Could you check a few things on this model? Use its own coordinates, in mm. A direction names the side the tool comes from. Give positions to 0.01 mm unless a question says otherwise; leave off trailing zeros. Order: outer loops, then holes, each group sorted by start corner. A loop starts at its lowest first (then second) coordinate and runs counter-clockwise, first axis right, second up. Notation, with made-up numbers: M 59,-5 L 66,-5 A8 cw 66,1 Z; hole C 84.25,56.5 d8. An arc over 180 degrees is marked long. Use a Markdown table: item, result. Add a question column.
```python
from build123d import *

# Parameters (mm, degrees)
F0_W     = 152.4
F0_H     = 152.4
F1_DEPTH = 12.7
F4_W     = 1828.8
F4_H     = 76.2
F5_DEPTH = 76.2
F6_W     = 114.3
F6_H     = 114.3
F6_W_2   = 76.2
F6_H_2   = 76.2
F7_DEPTH = 12.7
F8_W     = 114.3
F8_H     = 114.3
F9_DEPTH = 12.7


with BuildPart() as f1:
    # F0 (on Right) → F1 (new body)
    with BuildSketch(Plane.YZ):
        with Locations((4154.9873268127, -3903.1877601624)):
            Rectangle(F0_W, F0_H)
    extrude(amount=F1_DEPTH)


with BuildPart() as f1_1:
    # F2: moved
    add(f1.part.moved(Location((706.12, -1079.5, 1186.18))))


with BuildPart() as f5:
    # F4 (on Front) → F5 (new body)
    with BuildSketch(Plane.XZ):
        Rectangle(F4_W, F4_H)
    extrude(amount=F5_DEPTH)

    # F6 (on face) → F7 (join)
    with BuildSketch(Plane.YZ.offset(914.4)):
        with Locations((-38.1, 0)):
            Rectangle(F6_W, F6_H)
        with Locations((-38.1, 0)):
            Rectangle(F6_W_2, F6_H_2, mode=Mode.SUBTRACT)
        with Locations((-38.1, 0)):
            Rectangle(F6_W_2, F6_H_2)
    extrude(amount=F7_DEPTH)

    # F8 (on face) → F9 (join)
    with BuildSketch(Plane(origin=(-914.4, 0, 0), x_dir=(0, -1, 0), z_dir=(-1, 0, 0))):
        with Locations((38.1, 0)):
            Rectangle(F8_W, F8_H)
    extrude(amount=F9_DEPTH)


solid = f5.part
```
1) Suppose I cut it at B-B on y = -56. Please give me the cut outline in (x, z), and give its area (3 significant figures).
2) Suppose I cut it at A-A on z = -18. Please give me the cut outline in (x, y), and give its area (3 significant figures).
3) Suppose I cut it at C-C on x = -131. Please give me the cut outline in (y, z).
4) We'd pull the mould along X, two halves only. Please class faces 5 (the face through (927.1, -39, 1)), 6 (the face through (-13, -76.2, 1)), 7 (the face through (-927.1, -37, 1)): pulls with the +X half, pulls with the -X half, needs draft (parallel to the pull), parting line crosses it, or undercut.
5) For pin 1 (23 mm diameter, centred on x = 420, z = 5.5, fed in from +Y); pin 2 (4 mm diameter, centred on x = -29.5, z = 35.5, fed in from -Y); pin 3 (1.5 mm diameter, centred on x = 443.5, y = -39, fed in from -Z), each with a flat end and sliding along its axis, tell me the tip position at first contact or that it passes through.
6) Please list where these lines run through material, in increasing order: line 1 (X direction, y = -88.5, z = -4.5); line 2 (Z direction, x = 213.5, y = -68.5); line 3 (Y direction, x = 638, z = 10). Write a range as from..to.
7) For faces 1 (the face through (-13, -38, -38.1)), 2 (the face through (-13, -38, 38.1)), 3 (the face through (-914.4, 1, 1)), 4 (the face through (-13, 0, 1)), which set-ups out of +Z, -Z, +X, -X, +Y, -Y let a thin tool reach every point of the face, with its end or its side?
Values found:
| question | item | result |
|---|---|---|
| 1 | outline | M -927.1,-57.15 L -914.4,-57.15 L -914.4,-38.1 L 914.4,-38.1 L 914.4,-57.15 L 927.1,-57.15 L 927.1,57.15 L 914.4,57.15 L 914.4,38.1 L -914.4,38.1 L -914.4,57.15 L -927.1,57.15 Z |
| 1 | area | 142,000 mm^2 |
| 2 | outline | M -927.1,-95.25 L -914.4,-95.25 L -914.4,-76.2 L 914.4,-76.2 L 914.4,-95.25 L 927.1,-95.25 L 927.1,19.05 L 914.4,19.05 L 914.4,0 L -914.4,0 L -914.4,19.05 L -927.1,19.05 Z |
| 2 | area | 142,000 mm^2 |
| 3 | outline | M -76.2,-38.1 L 0,-38.1 L 0,38.1 L -76.2,38.1 Z |
| 4 | face 5 | pulls with the +X half |
| 4 | face 6 | undercut |
| 4 | face 7 | pulls with the -X half |
| 5 | pin 1 | stops at y = 0 |
| 5 | pin 2 | stops at y = -76.2 |
| 5 | pin 3 | stops at z = -38.1 |
| 6 | line 1 | x = -927.1..-914.4, 914.4..927.1 |
| 6 | line 2 | z = -38.1..38.1 |
| 6 | line 3 | y = -76.2..0 |
| 7 | face 1 | -Z, +Y, -Y |
| 7 | face 2 | +Z, +Y, -Y |
| 7 | face 3 | none |
| 7 | face 4 | +Z, -Z, +Y |
